Could you check a few things on this model? Use its own coordinates, in mm. Coordinates: 2 decimals unless noted, no trailing zeros. Write each loop counter-clockwise with the first axis right and the second up, starting at its lowest first coordinate (ties: lowest second). Pieces come first, ordered by that corner, then holes. Notation, with made-up numbers: (65.5, 73) - (100.5, 73) arc R32 ccw to (100.5, 111) - close; hole circle Ø2 at (65.5, -0.75). An arc over 180 degrees is marked (long way). Answer as a JSON object with one key per item and string values. Group by question number.
1) If we section it at B-B (x = -27.5): Write out the boundary of the cut face in (y, z).
2) If we section it at A-A (x = 40.5): Write out the boundary of the cut face in (y, z).
3) Will these pins go through, and if not, where does the flat tip stop? pin 1 Ø12 at (y, z) = (-38.5, -4) entering from +X; pin 2 Ø6 at (x, y) = (-38, -37.5) entering from +Z; pin 3 Ø12 at (x, z) = (-39.5, -7) entering from +Y.
4) Please list where these lines run through material, in increasing order: line 1 along X through (y, z) = (-36, -5.25); line 2 along X through (y, z) = (-58.5, -2); line 3 along Y through (x, z) = (13, -4.75).
```python
from build123d import *

# Parameters (mm, degrees)
F1_DEPTH = 7
F2_ANGLE = -10
F3_W     = 126.412388
F3_H     = 62.651056
F4_DEPTH = 25


with BuildPart() as f1:
    # F0 (on Top) → F1 (new body)
    with BuildSketch(Plane.XY):
        with BuildLine():
            ThreePointArc((16.768167, 4.455454), (0, -17.35), (-16.768167, 4.455454))
            ThreePointArc((-16.768167, 4.455454), (-16.904061, 5.67856), (-17.829723, 6.489489))
            Line((-17.829723, 6.489489), (-19.581941, 7.127244))
            ThreePointArc((-19.581941, 7.127244), (-20.860413, 7.046862), (-21.670162, 6.054261))
            ThreePointArc((-21.670162, 6.054261), (-21.640699, -6.158747), (-15.235151, -16.557179))
            ThreePointArc((-15.235151, -16.557179), (-13.719641, -21.22611), (-16.927946, -24.941278))
            ThreePointArc((-16.927946, -24.941278), (-40.904751, -43.234384), (-50, -71.988538))
            Line((-50, -71.988538), (-43.59892, -71.988538))
            ThreePointArc((-43.59892, -71.988538), (0, -28.389618), (43.59892, -71.988538))
            Line((43.59892, -71.988538), (50, -71.988538))
            ThreePointArc((50, -71.988538), (40.904751, -43.234384), (16.927946, -24.941278))
            ThreePointArc((16.927946, -24.941278), (13.719641, -21.22611), (15.235151, -16.557179))
            ThreePointArc((15.235151, -16.557179), (21.640699, -6.158747), (21.670162, 6.054261))
            ThreePointArc((21.670162, 6.054261), (20.860413, 7.046862), (19.581941, 7.127244))
            Line((19.581941, 7.127244), (17.829723, 6.489489))
            ThreePointArc((17.829723, 6.489489), (16.904061, 5.67856), (16.768167, 4.455454))
        make_face()
    extrude(amount=F1_DEPTH)


with BuildPart() as f1_1:
    # F2: moved
    add(f1.part.rotate(Axis((-46.79946, -71.988538, 7), (1, 0, 0)), F2_ANGLE))


with BuildPart() as f4:
    # F3 (on Front) → F4 (new body)
    with BuildSketch(Plane.XZ):
        with Locations((-1.744712, 3.013594)):
            Rectangle(F3_W, F3_H)
    extrude(amount=F4_DEPTH)


with BuildPart() as f4_1:
    # F5: moved
    add(f4.part.moved(Location((0, -71.85045, 0))))


with BuildPart() as f1_2:
    add(f1_1.part)

    # F6: cut F4
    add(f4_1.part, mode=Mode.SUBTRACT)


solid = f1_2.part
```
Here are the results:
{
 "1": {"outline": "(-39.89, -5.77) - (-32.08, -7.14) - (-30.86, -0.25) - (-38.67, 1.13) - close"},
 "2": {"outline": "(-57.31, -2.7) - (-44.33, -4.99) - (-43.11, 1.91) - (-56.09, 4.2) - close"},
 "3": {"pin 1": "stops at x = 40.81", "pin 2": "stops at z = 1.45", "pin 3": "stops at y = -36.67"},
 "4": {"line 1": "x = -32.99 to -22.12, 22.12 to 32.99", "line 2": "x = -47.74 to -40.99, 40.99 to 47.74", "line 3": "y = -31.8 to -12.63"}
}
